```python
from build123d import *

# Parameters (mm, degrees)
EXTRUDE_1_DEPTH     = 20
SKETCH_2_R          = 14
CUT_EXTRUDE_1_DEPTH = 8
SKETCH_3_R          = 12
CUT_EXTRUDE_2_DEPTH = 218.644205069
SKETCH_4_R          = 5.5
CUT_EXTRUDE_3_DEPTH = 219.231528428
SKETCH_6_R          = 3.3
CUT_EXTRUDE_4_DEPTH = 219.231528428


with BuildPart() as part:
    # 草图1 → 凸台-拉伸1 (new body)
    with BuildSketch(Plane.XY):
        with BuildLine():
            Line((0, 85), (200, 85))
            Line((200, 85), (200, -85))
            Line((200, -85), (0, -85))
            ThreePointArc((0, -85), (-85, 0), (0, 85))
        make_face()
    extrude(amount=EXTRUDE_1_DEPTH)

    # 草图2 → 切除-拉伸1 (cut)
    with BuildSketch(Plane.XY.offset(20)):
        Circle(SKETCH_2_R)
    extrude(amount=-CUT_EXTRUDE_1_DEPTH, mode=Mode.SUBTRACT)

    # 草图3 → 切除-拉伸2 (cut, through all)
    with BuildSketch(Plane.XY.offset(12)):
        Circle(SKETCH_3_R)
    extrude(amount=-CUT_EXTRUDE_2_DEPTH, mode=Mode.SUBTRACT)

    # 草图4 → 切除-拉伸3 (cut, through all)
    with BuildSketch(Plane.XY.offset(20)):
        with Locations((-72.5, 0)):
            Circle(SKETCH_4_R)
        with Locations((36.25, 62.786841774)):
            Circle(SKETCH_4_R)
        with Locations((36.25, -62.786841774)):
            Circle(SKETCH_4_R)
    extrude(amount=-CUT_EXTRUDE_3_DEPTH, mode=Mode.SUBTRACT)

    # 草图6 → 切除-拉伸4 (cut, through all)
    with BuildSketch(Plane.XY.offset(20)):
        with Locations((47.3, 13)):
            Circle(SKETCH_6_R)
        with Locations((47.3, -13)):
            Circle(SKETCH_6_R)
    extrude(amount=-CUT_EXTRUDE_4_DEPTH, mode=Mode.SUBTRACT)


solid = part.part
```
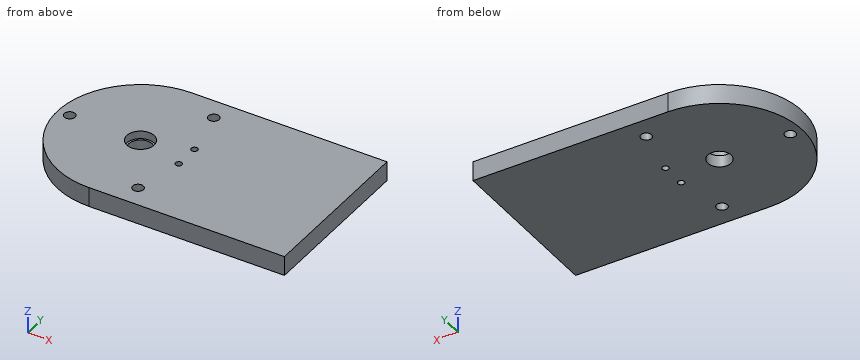
Source: CAD feature listing. Evaluate the final solid. Frame: model axes, mm. Give positions to 0.01 mm unless a question says otherwise; leave off trailing zeros. Order: outer loops, then holes, each group sorted by start corner. A loop starts at its lowest first (then second) coordinate and runs counter-clockwise, first axis right, second up.
(1) Contact query for a flat-ended pin moving along its axis: P1, Ø4, axis at y = 24.5, z = 9, coming from the -X side. Output: stop coordinate, or through.
(2) Section query B-B (x = 3). Return the cut outline in (y, z), plus the area to 3 significant figures.
(3) Material intervals for line 1 along Y through (x, z) = (36.25, 10.5); line 2 along Y through (x, z) = (0, 16.25); line 3 along Y through (x, z) = (0, 4), sorted ascending.
(4) Section query A-A (x = 47.3). Return the cut outline in (y, z), plus the area to 3 significant figures.
(5) Section query C-C (x = -72.5). Return the cut outline in (y, z), plus the area to 3 significant figures.
Outcome:
1. P1: stops at x = -81.97
2. outline: (-85, 0) - (-11.62, 0) - (-11.62, 12) - (-13.67, 12) - (-13.67, 20) - (-85, 20) - close; (11.62, 0) - (85, 0) - (85, 20) - (13.67, 20) - (13.67, 12) - (11.62, 12) - close
2. area: 2,900 mm2
3. line 1: y = -85 to -68.29, -57.29 to 57.29, 68.29 to 85
3. line 2: y = -85 to -14, 14 to 85
3. line 3: y = -85 to -12, 12 to 85
4. outline: (-85, 0) - (-16.3, 0) - (-16.3, 20) - (-85, 20) - close; (-9.7, 0) - (9.7, 0) - (9.7, 20) - (-9.7, 20) - close; (16.3, 0) - (85, 0) - (85, 20) - (16.3, 20) - close
4. area: 3,140 mm2
5. outline: (-44.37, 0) - (-5.5, 0) - (-5.5, 20) - (-44.37, 20) - close; (5.5, 0) - (44.37, 0) - (44.37, 20) - (5.5, 20) - close
5. area: 1,550 mm2
